from build123d import *

# Parameters (mm, degrees)
SKETCH2_R           = 3.425
BOSS_EXTRUDE2_DEPTH = 3
SKETCH3_W           = 133.4
SKETCH3_H           = 12.75
CUT_EXTRUDE1_DEPTH  = 351.642267846


with BuildPart() as part:
    # Sketch2 → Boss-Extrude2 (new body)
    with BuildSketch(Plane.XY):
        with BuildLine():
            Line((25.03035901, 0), (111.286489227, 49.8))
            ThreePointArc((111.286489227, 49.8), (152.858332199, 69.766604349), (181.6, 33.7))
            Line((181.6, 33.7), (181.6, 0))
            Line((181.6, 0), (315, 0))
            Line((315, 0), (315, 145))
            Line((315, 145), (38, 145))
            Line((38, 145), (38, 154))
            Line((38, 154), (19, 154))
            Line((19, 154), (0, 154))
            Line((0, 154), (0, 0))
            Line((0, 0), (25.03035901, 0))
        make_face()
        with Locations((19, 135)):
            Circle(SKETCH2_R, mode=Mode.SUBTRACT)
    extrude(amount=BOSS_EXTRUDE2_DEPTH)

    # Sketch3 → Cut-Extrude1 (cut, through all)
    with BuildSketch(Plane.XY.offset(3)):
        with Locations((248.3, 6.375)):
            Rectangle(SKETCH3_W, SKETCH3_H)
    extrude(amount=-CUT_EXTRUDE1_DEPTH, mode=Mode.SUBTRACT)


solid = part.part
Work out the finished part from the listing and answer in its coordinate system (mm). A direction names the side the tool comes from. Round coordinates to 2 decimals unless told otherwise and drop trailing zeros. Loops run counter-clockwise (first coordinate to the right, second up) from the corner with the lowest first, then second, coordinate; pieces in that order, holes last. Notation, with made-up numbers: (81.25, -6.75) - (90.25, -6.75) arc R13 cw to (90.25, 14.25) - close; hole circle Ø11 at (-27, -8.5). An arc over 180 degrees is marked (long way). Use one line per item in the form item = value. Start each with the question number.
(1) Find section D-D on x = 230. Determine the outline of the cut face in (y, z).
(2) Which of the six approach directions +Z, -Z, +X, -X, +Y, -Y give full straight-line access (tool end or side, diameter ignored) to faces 3 (the face through (67.55, 24.55, 1.48)), 4 (the face through (18.6, 138.4, 1.5))?
(3) Consider line 1 (Y direction, x = 19, z = 1) (3 decimals); line 2 (X direction, y = 135, z = 1.65) (3 decimals); line 3 (Y direction, x = 269.5, z = 0.8). Determine where each line is inside the solid, lowest interval first.
(4) Find section B-B on y = 135. Determine the outline of the cut face in (x, z) (3 decimals).
(5) Flat-ended cylindrical pins translate along their axes: P1, Ø1.5, axis at x = 183.5, z = 2, coming from the +Y side; P2, Ø6, axis at x = 19, y = 135, coming from the -Z side; P3, Ø0.9, axis at x = 225, z = 1.5, coming from the -Y side. Find the tip coordinate at first contact, or state that the pin passes through.
(6) Determine the mould class of faces 1 (the face through (152.177, 69.916, 1.479)), 2 (the face through (155, 78, 0)) for opening direction X: +X half, -X half, draft (parallel to the pull), parting line (faces both ways), or undercut.
(7) Find section C-C on z = 2.1. Determine the outline of the cut face in (x, y) (3 decimals), and give its area (3 significant figures).
(8) Find section A-A on x = 19. Determine the outline of the cut face in (y, z) (3 decimals).
Answer list:
q1.outline = (12.75, 0) - (145, 0) - (145, 3) - (12.75, 3) - close
q2.face_3 = +Z, -Z, -Y
q2.face_4 = +Z, -Z
q3.line_1 = 0 to 131.575, 138.425 to 154
q3.line_2 = 0 to 15.575, 22.425 to 315
q3.line_3 = 12.75 to 145
q4.outline = (0, 0) - (15.575, 0) - (15.575, 3) - (0, 3) - close; (22.425, 0) - (315, 0) - (315, 3) - (22.425, 3) - close
q5.P1 = 145
q5.P2 = through
q5.P3 = 12.75
q6.face_1 = undercut
q6.face_2 = draft
q7.outline = (0, 0) - (25.03, 0) - (111.286, 49.8) arc R37 cw to (181.6, 33.7) - (181.6, 12.75) - (315, 12.75) - (315, 145) - (38, 145) - (38, 154) - (0, 154) - close; hole circle Ø6.85 at (19, 135)
q7.area = 37,700 mm^2
q8.outline = (0, 0) - (131.575, 0) - (131.575, 3) - (0, 3) - close; (138.425, 0) - (154, 0) - (154, 3) - (138.425, 3) - close
